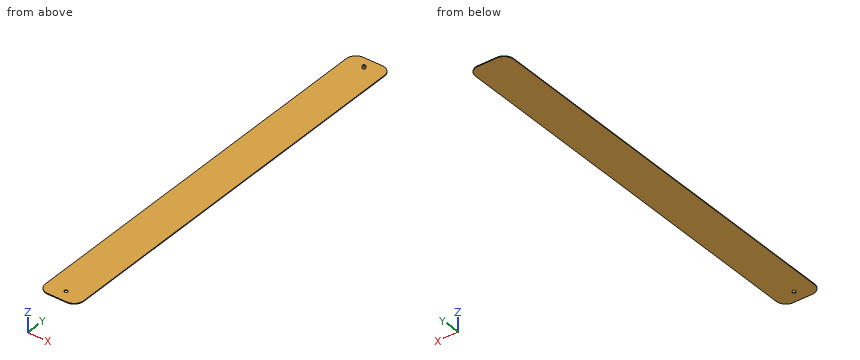
```python
from build123d import *

# Parameters (mm, degrees)
F1_DEPTH = 0.4
F2_R     = 0.75
F3_DEPTH = 1.5
F3_TAPER = -3
F5_D     = 1.8


# Not quite as in the source:
# - a fillet or chamfer that OpenCascade refuses, or shapes differently, is made with other operations: its cross-section is extruded or revolved along the edge and cut away or added


with BuildPart() as f1:
    # F0 (on Top) → F1 (new body)
    with BuildSketch(Plane.XY):
        with BuildLine():
            Line((-6.5418671444, 67.6613259315), (-16.5418671444, 67.6613259315))
            ThreePointArc((-16.5418671444, 67.6613259315), (-20.0774010503, 66.1968598375), (-21.5418671444, 62.6613259315))
            Line((-21.5418671444, 62.6613259315), (-21.5418671444, -142.3386740685))
            ThreePointArc((-21.5418671444, -142.3386740685), (-20.0774010503, -145.8742079744), (-16.5418671444, -147.3386740685))
            Line((-16.5418671444, -147.3386740685), (-6.5418671444, -147.3386740685))
            ThreePointArc((-6.5418671444, -147.3386740685), (-3.0063332385, -145.8742079744), (-1.5418671444, -142.3386740685))
            Line((-1.5418671444, -142.3386740685), (-1.5418671444, 62.6613259315))
            ThreePointArc((-1.5418671444, 62.6613259315), (-3.0063332385, 66.1968598375), (-6.5418671444, 67.6613259315))
        make_face()
    extrude(amount=F1_DEPTH)

    # F2 (on face) → F3 (join)
    with BuildSketch(Plane.XY.offset(0.4)):
        with Locations((-11.5418671444, 61.6613259315)):
            Circle(F2_R)
    extrude(amount=F3_DEPTH, taper=F3_TAPER)

    # F4: chamfer of 0.4 on 1 edges, made by hand

    # F4_s1 → F4_t2 (revolve, cut)
    with BuildSketch(Plane.XZ.offset(-61.6613259315)):
        Polygon((-10.734189858, 1.5005481861), (-11.1132554755, 1.9), (-10.7132554755, 1.9), align=None)
    revolve(axis=Axis((-11.5418671444, 61.6613259315, 1.9), (0, 0, -1)), mode=Mode.SUBTRACT)

    # F5 (through all)
    with Locations(Plane.XY.offset(0.4)):
        with Locations((-11.5418671444, -141.3386740685)):
            Hole(F5_D / 2)


solid = f1.part
```
Verification items for the finished model (mm, model axes). Round coordinates to 2 decimals unless told otherwise and drop trailing zeros. Loops run counter-clockwise (first coordinate to the right, second up) from the corner with the lowest first, then second, coordinate; pieces in that order, holes last. Notation, with made-up numbers: (14, -14) -> (36, -14) arc R26 ccw to (36, 13) -> close; hole circle Ø8 at (-29, 64). An arc over 180 degrees is marked (long way). Answer as a JSON object with one key per item and string values.
Q1. Section check B-B (z = 0.85). Record the boundary of the cut face in (x, y).
Data:
{"outline": "circle Ø1.55 at (-11.54, 61.66)"}
Q2. Section check C-C (x = -4.25). Record the boundary of the cut face in (y, z).
Data:
{"outline": "(-146.78, 0) -> (67.11, 0) -> (67.11, 0.4) -> (-146.78, 0.4) -> close"}
Q3. Go/stop test with flat-tipped pins: P1, Ø8, axis at x = -11.5, y = -34, coming from the -Z side; P2, Ø10, axis at x = -10, y = -120, coming from the +Z side. Record where each tip stops, or that it passes through.
Data:
{"P1": "stops at z = 0", "P2": "stops at z = 0.4"}
Q4. Section check A-A (y = 39). Record the boundary of the cut face in (x, z), then the cut area to 3 significant figures.
Data:
{"outline": "(-21.54, 0) -> (-1.54, 0) -> (-1.54, 0.4) -> (-21.54, 0.4) -> close", "area": "8.00 mm2"}
Q5. Scan lines: line 1 (Z direction, x = -20.25, y = -78.5); line 2 (Y direction, x = -12, z = 0.65). Record each from-to range of solid material in increasing order. Write a range as from..to.
Data:
{"line 1": "z = 0..0.4", "line 2": "y = 61.05..62.27"}
